Here's how the part is built. I have some questions about the finished solid (model axes, mm). Face numbers are marked on the shaded views. A direction names the side the tool comes from. Coordinates: 2 decimals unless noted, no trailing zeros. Loops run counter-clockwise (first coordinate to the right, second up) from the corner with the lowest first, then second, coordinate; pieces in that order, holes last. Notation, with made-up numbers: (79, 18) -> (118, 18) arc R18 ccw to (118, 44) -> close; hole circle Ø1 at (67.25, 51). An arc over 180 degrees is marked (long way). Use CSV: the item, a comma, the result in double quotes. Start each with the question number.
from build123d import *

# Parameters (mm, degrees)
SKETCH1_W           = 90
SKETCH1_H           = 100
BOSS_EXTRUDE1_DEPTH = 40
SHELL1_T            = -3
FILLET1_R           = 10
FILLET2_R           = 10
FILLET3_R           = 10
FILLET4_R           = 10


with BuildPart() as part:
    # Sketch1 → Boss-Extrude1 (new body)
    with BuildSketch(Plane(origin=(0, 0, 0), x_dir=(1, 0, 0), z_dir=(0, 1, 0))):
        with Locations((36.913730494, -32.688282622)):
            Rectangle(SKETCH1_W, SKETCH1_H)
    extrude(amount=BOSS_EXTRUDE1_DEPTH)

    # Shell1
    shell1_openings = [part.faces().sort_by_distance(p)[0] for p in [
        (36.913730494, 0, 32.688282622),
    ]]
    offset(amount=SHELL1_T, openings=shell1_openings, kind=Kind.INTERSECTION)

    # Fillet1
    fillet1_edges = [part.edges().sort_by_distance(p)[0] for p in [
        (81.913730494, 20, 82.688282622),
    ]]
    fillet(fillet1_edges, radius=FILLET1_R)

    # Fillet2
    fillet2_edges = [part.edges().sort_by_distance(p)[0] for p in [
        (-8.086269506, 20, 82.688282622),
    ]]
    fillet(fillet2_edges, radius=FILLET2_R)

    # Fillet3
    fillet3_edges = [part.edges().sort_by_distance(p)[0] for p in [
        (81.913730494, 20, -17.311717378),
    ]]
    fillet(fillet3_edges, radius=FILLET3_R)

    # Fillet4
    fillet4_edges = [part.edges().sort_by_distance(p)[0] for p in [
        (-8.086269506, 20, -17.311717378),
    ]]
    fillet(fillet4_edges, radius=FILLET4_R)


solid = part.part
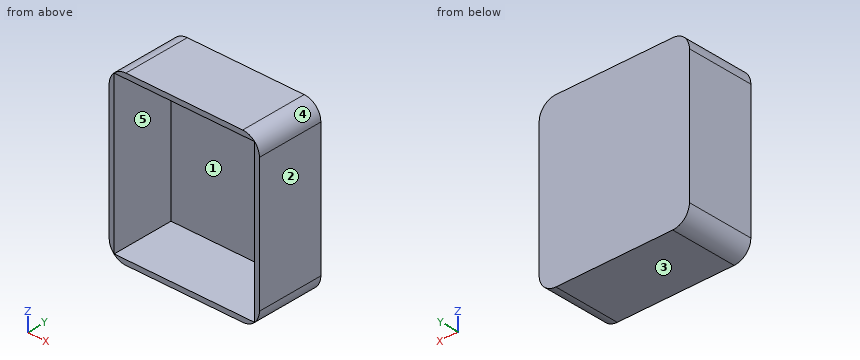
1) Which directions (+Z, -Z, +X, -X, +Y, -Y) give clear straight access to the entire face, cutting with the end or side of a thin tool? Please do the marked faces 4 and 5.
2) I want a section at B-B, the plane x = 27.5. Please give me the cut outline in (y, z).
3) I want a section at A-A, the plane y = 32.5. Please give me the cut outline in (x, z), plus the area to 3 significant figures.
4) I want a section at C-C, the plane z = -6. Please give me the cut outline in (x, y), plus the area to 3 significant figures.
5) Thinking about a two-plate mould opening in X: for the marked faces 1, 2 and 3, which applies, pulls with the +X half, pulls with the -X half, needs draft (parallel to the pull), parting line crosses it, or undercut?
6) Please list where these lines run through material, in increasing order: L1, parallel to Z at x = 54, y = 36; L2, parallel to X at y = 32.5, z = 54.5; L3, parallel to Y at x = 1.5, z = -11.5. Write a range as [from, to].
7) For P1, Ø3, axis at x = 32.5, z = 53, coming from the -Y side, with a flat end and sliding along its axis, tell me the tip position at first contact or that it passes through.
Return value:
1,face 4,"+Z, +X, +Y, -Y"
1,face 5,"-Y"
2,outline,"(0, -17.31) -> (40, -17.31) -> (40, 82.69) -> (0, 82.69) -> (0, 79.69) -> (37, 79.69) -> (37, -14.31) -> (0, -14.31) -> close"
3,outline,"(-8.09, -7.31) arc R10 ccw to (1.91, -17.31) -> (71.91, -17.31) arc R10 ccw to (81.91, -7.31) -> (81.91, 72.69) arc R10 ccw to (71.91, 82.69) -> (1.91, 82.69) arc R10 ccw to (-8.09, 72.69) -> close; hole (-5.09, -14.31) -> (78.91, -14.31) -> (78.91, 79.69) -> (-5.09, 79.69) -> close"
3,area,"1,020 mm²"
4,outline,"(-8.09, 0) -> (-5.09, 0) -> (-5.09, 37) -> (78.91, 37) -> (78.91, 0) -> (81.91, 0) -> (81.91, 40) -> (-8.09, 40) -> close"
4,area,"492 mm²"
5,face 1,"undercut"
5,face 2,"pulls with the +X half"
5,face 3,"needs draft"
6,L1,"z = [-17.31, -14.31], [79.69, 82.69]"
6,L2,"x = [-8.09, -5.09], [78.91, 81.91]"
6,L3,"y = [37, 40]"
7,P1,"stops at y = 37"
